from build123d import *

# Parameters (mm, degrees)
F0_R     = 10
F1_DEPTH = 25


with BuildPart() as f1:
    # F0 (on Front) → F1 (new body)
    with BuildSketch(Plane.XZ):
        with BuildLine():
            ThreePointArc((4.105443, 24.660603), (19.074015, 16.161125), (25, 0))
            ThreePointArc((25, 0), (18.40534, -16.918731), (2.100523, -24.9116))
            Line((2.100523, -24.9116), (90, -17.5))
            ThreePointArc((90, -17.5), (72.51488, 0.721517), (91.441807, 17.440504))
            Line((91.441807, 17.440504), (4.105443, 24.660603))
        make_face()
        with BuildLine():
            Line((0, 25), (4.105443, 24.660603))
            ThreePointArc((4.105443, 24.660603), (2.059724, 24.915006), (0, 25))
        make_face()
        with BuildLine():
            ThreePointArc((107.5, 0), (102.874036, 11.853657), (91.441807, 17.440504))
            ThreePointArc((91.441807, 17.440504), (72.51488, 0.721517), (90, -17.5))
            ThreePointArc((90, -17.5), (102.374369, -12.374369), (107.5, 0))
        make_face()
        with Locations((90, 0)):
            Circle(F0_R, mode=Mode.SUBTRACT)
        Circle(F0_R)
        with BuildLine():
            ThreePointArc((2.100523, -24.9116), (18.40534, -16.918731), (25, 0))
            ThreePointArc((25, 0), (19.074015, 16.161125), (4.105443, 24.660603))
            Line((4.105443, 24.660603), (0, 25))
            ThreePointArc((0, 25), (-24.97789, -1.051191), (2.100523, -24.9116))
        make_face()
        Circle(F0_R, mode=Mode.SUBTRACT)
    extrude(amount=F1_DEPTH)


solid = f1.part
Could you check a few things on this model? Use its own coordinates, in mm. Give positions to 0.01 mm unless a question says otherwise; leave off trailing zeros. Loops run counter-clockwise (first coordinate to the right, second up) from the corner with the lowest first, then second, coordinate; pieces in that order, holes last. Notation, with made-up numbers: (-34.5, 11) -> (-13.5, 11) arc R21 cw to (-13.5, 37) -> close; hole circle Ø1 at (18, -28.5). An arc over 180 degrees is marked (long way). Answer as CSV lines item,"result". Start each with the question number.
(1) I need wall thicknesses on probe 1 along X at (y, z) = (-6, -8); probe 2 along X at (y, z) = (-5.5, 5); probe 3 along Z at (x, y) = (90, -11). Which ranges of each line are inside material? Lowest first, please.
(2) If we section it at D-D on z = 5.5: Write out the boundary of the cut face in (x, y), then the cut area to 3 significant figures.
(3) If we section it at C-C on x = -2.5: Write out the boundary of the cut face in (y, z), then the cut area to 3 significant figures.
(4) If we section it at B-B on y = -22: Write out the boundary of the cut face in (x, z).
(5) I'm going to push flat-ended pins straight in: pin 1 Ø12 at (y, z) = (-14.5, 8.5) entering from +X; pin 2 Ø1 at (y, z) = (-5.5, 16) entering from +X; pin 3 Ø3 at (y, z) = (-6, 12) entering from +X; pin 4 Ø23 at (x, z) = (90, 0) entering from +Y. Where does each tip first touch, or does it pass through?
(6) If we section it at A-A on z = -6.5: Write out the boundary of the cut face in (x, y), then the cut area to 3 significant figures.
(7) We'd pull the mould along X, two halves only. Please class faces 1 (the cylindrical face through (80, -12, 0)), 2 (the flat face through (40, 0, 0)), 3 (the flat face through (45.43, -12.32, -21.26)): released by +X, released by -X, zero draft, split by the parting line, or undercut.
Computed:
1,probe 1,"x = -23.69 to -6, 6 to 84, 96 to 105.56"
1,probe 2,"x = -24.49 to -8.66, 8.66 to 81.34, 98.66 to 106.77"
1,probe 3,"z = -17.5 to -10, 10 to 17.56"
2,outline,"(-24.39, -25) -> (-8.35, -25) -> (-8.35, 0) -> (-24.39, 0) -> close; (8.35, -25) -> (81.65, -25) -> (81.65, 0) -> (8.35, 0) -> close; (98.35, -25) -> (106.61, -25) -> (106.61, 0) -> (98.35, 0) -> close"
2,area,"2,440 mm2"
3,outline,"(-25, -24.87) -> (0, -24.87) -> (0, -9.68) -> (-25, -9.68) -> close; (-25, 9.68) -> (0, 9.68) -> (0, 24.87) -> (-25, 24.87) -> close"
3,area,"760 mm2"
4,outline,"(0, 25) arc R25 ccw (long way) to (2.1, -24.91) -> (90, -17.5) arc R17.5 ccw to (107.5, 0) arc R17.5 ccw to (91.44, 17.44) -> (4.11, 24.66) arc R25 ccw to start; hole circle Ø20 at (0, 0); hole circle Ø20 at (90, 0)"
5,pin 1,"stops at x = 107.32"
5,pin 2,"stops at x = 98.12"
5,pin 3,"stops at x = 104"
5,pin 4,"stops at y = 0"
6,outline,"(-24.14, -25) -> (-7.6, -25) -> (-7.6, 0) -> (-24.14, 0) -> close; (7.6, -25) -> (82.4, -25) -> (82.4, 0) -> (7.6, 0) -> close; (97.6, -25) -> (106.25, -25) -> (106.25, 0) -> (97.6, 0) -> close"
6,area,"2,500 mm2"
7,face 1,"undercut"
7,face 2,"zero draft"
7,face 3,"released by +X"
